Work out the finished part from the listing and answer in its coordinate system (mm). Face numbers are marked on the shaded views. Give positions to 0.01 mm unless a question says otherwise; leave off trailing zeros. Loops run counter-clockwise (first coordinate to the right, second up) from the corner with the lowest first, then second, coordinate; pieces in that order, holes last. Notation, with made-up numbers: (77, -25.75) - (117, -25.75) arc R21 ccw to (117, -13.75) - close; hole circle Ø2 at (1, 69). An arc over 180 degrees is marked (long way). One line per question, with ' | ' between items. Start each with the question number.
1. Section B-B (y = 67.5) is taken. Determine the outline of the cut face in (x, z), plus the area to 3 significant figures.
2. Section A-A (z = 0) is taken. Determine the outline of the cut face in (x, y).
3. Find the intervals of material crossed by line 1 (X direction, y = 123, z = 0); line 2 (X direction, y = 100, z = 0), in increasing order.
4. Each of these flat-tipped pins is pushed along its axis until it touches: pin 1 (1.5 mm diameter, centred on y = 116.5, z = 39, fed in from -X); pin 2 (24.5 mm diameter, centred on y = 101.5, z = 18.5, fed in from -X); pin 3 (4 mm diameter, centred on x = -14, z = -34, fed in from +Y). Where does it stop, or does it pass through?
5. For a pull along Z with two mould halves and no side action, classify the marked faces 1, 2 and 3 as released by +Z, released by -Z, zero draft, split by the parting line, or undercut.
6. Section C-C (y = 18.5) is taken. Determine the outline of the cut face in (x, z), plus the area to 3 significant figures.
7. Section D-D (y = 45.5) is taken. Determine the outline of the cut face in (x, z), plus the area to 3 significant figures.
from build123d import *

# Parameters (mm, degrees)
SKETCH1_R           = 55
BOSS_EXTRUDE1_DEPTH = 150
FILLET1_R           = 10
SKETCH3_R           = 42.5
CUT_EXTRUDE2_DEPTH  = 85
SKETCH13_R          = 42.5
BOSS_EXTRUDE3_DEPTH = 120


with BuildPart() as part:
    # Sketch1 → Boss-Extrude1 (new body)
    with BuildSketch(Plane(origin=(0, 0, 0), x_dir=(1, 0, 0), z_dir=(0, 1, 0))):
        Circle(SKETCH1_R)
    extrude(amount=BOSS_EXTRUDE1_DEPTH)

    # Fillet1
    fillet1_edges = [part.edges().sort_by_distance(p)[0] for p in [
        (-55, 0, 0),
    ]]
    fillet(fillet1_edges, radius=FILLET1_R)

    # Sketch3 → Cut-Extrude2 (cut)
    with BuildSketch(Plane(origin=(0, 150, 0), x_dir=(1, 0, 0), z_dir=(0, 1, 0))):
        Circle(SKETCH3_R)
    extrude(amount=-CUT_EXTRUDE2_DEPTH, mode=Mode.SUBTRACT)

    # Sketch13 → Boss-Extrude3 (add)
    with BuildSketch(Plane(origin=(0, 0, 0), x_dir=(0, 0, -1), z_dir=(1, 0, 0))):
        with Locations((0, 71.359942757)):
            Circle(SKETCH13_R)
    extrude(amount=BOSS_EXTRUDE3_DEPTH)


solid = part.part
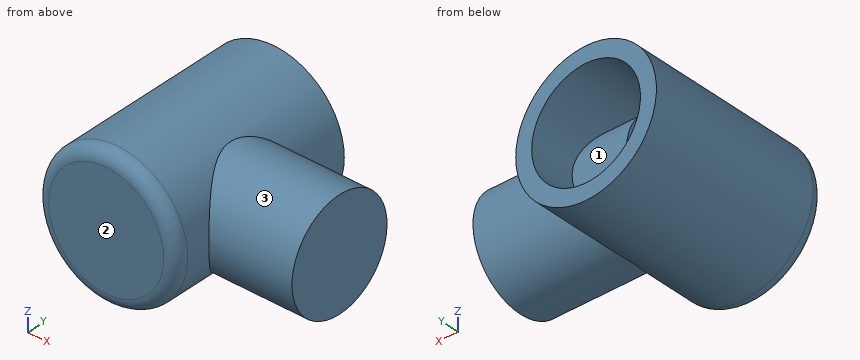
Conclusion:
1) outline: (35.12, -42.32) - (120, -42.32) - (120, 42.32) - (35.12, 42.32) arc R55 ccw (long way) to start; hole (0, -42.32) - (0, 42.32) - (3.86, 42.32) arc R42.5 ccw (long way) to (3.86, -42.32) - close | area: 12,700 mm²
2) outline: (-55, 10) arc R10 ccw to (-45, 0) - (45, 0) arc R10 ccw to (55, 10) - (55, 28.86) - (120, 28.86) - (120, 113.86) - (55, 113.86) - (55, 150) - (42.5, 150) - (42.5, 113.86) - (0, 113.86) - (0, 65) - (-42.5, 65) - (-42.5, 150) - (-55, 150) - close
3) line 1: -55 to -42.5, 42.5 to 55 | line 2: -55 to -42.5, 0 to 120
4) pin 1: x = -39.52 | pin 2: x = -54.64 | pin 3: y = 65
5) face 1: undercut | face 2: zero draft | face 3: split by the parting line
6) outline: circle Ø110 at (0, 0) | area: 9,500 mm²
7) outline: (43.45, -33.73) - (120, -33.73) - (120, 33.73) - (43.45, 33.73) arc R55 ccw (long way) to start | area: 14,100 mm²
